Autodesk Fusion 360 part; units mm, degrees
sketch "Sketch1" plane through (0, 0, 0) normal (0, 0, 1) x (1, 0, 0)
  line L0 (-50.4372, 47.8193) -> (49.5628, 47.8193)
  line L1 (49.5628, 47.8193) -> (49.5628, -63.1807)
  line L2 (49.5628, -63.1807) -> (-50.4372, -63.1807)
  line L3 (-50.4372, -63.1807) -> (-50.4372, 47.8193)
  line L4 (-18.6372, -27.5802) -> (-23.0372, -27.5802)
  line L5 (-23.0372, -27.5802) -> (-23.0372, -24.2802)
  line L6 (-23.0372, -24.2802) -> (-18.6372, -24.2802)
  line L7 (-18.6372, -24.2802) -> (-18.6372, -27.5802)
  line L8 (17.6628, -24.0807) -> (22.0628, -24.0807)
  line L9 (22.0628, -24.0807) -> (22.0628, -27.3807)
  line L10 (22.0628, -27.3807) -> (17.6628, -27.3807)
  line L11 (17.6628, -27.3807) -> (17.6628, -24.0807)
  line L12 (17.8378, -44.4057) -> (22.2378, -44.4057)
  line L13 (22.2378, -44.4057) -> (22.2378, -47.7057)
  line L14 (22.2378, -47.7057) -> (17.8378, -47.7057)
  line L15 (17.8378, -47.7057) -> (17.8378, -44.4057)
  line L16 (27.9628, -34.1807) -> (32.3628, -34.1807)
  line L17 (32.3628, -34.1807) -> (32.3628, -37.4807)
  line L18 (32.3628, -37.4807) -> (27.9628, -37.4807)
  line L19 (27.9628, -37.4807) -> (27.9628, -34.1807)
  line L20 (-33.0372, -34.1807) -> (-28.6372, -34.1807)
  line L21 (-28.6372, -34.1807) -> (-28.6372, -37.4807)
  line L22 (-28.6372, -37.4807) -> (-33.0372, -37.4807)
  line L23 (-33.0372, -37.4807) -> (-33.0372, -34.1807)
  line L24 (-13.0372, -34.1807) -> (-8.6372, -34.1807)
  line L25 (-8.6372, -34.1807) -> (-8.6372, -37.4807)
  line L26 (-8.6372, -37.4807) -> (-13.0372, -37.4807)
  line L27 (-13.0372, -37.4807) -> (-13.0372, -34.1807)
  line L28 (-23.4439, -44.4057) -> (-19.0439, -44.4057)
  line L29 (-19.0439, -44.4057) -> (-19.0439, -47.7057)
  line L30 (-19.0439, -47.7057) -> (-23.4439, -47.7057)
  line L31 (-23.4439, -47.7057) -> (-23.4439, -44.4057)
  dimension "d1" = 100
  dimension "d2" = 111
  dimension "d3" = 4.4
  dimension "d4" = 3.3
  dimension "d5" = 4.4
  dimension "d6" = 3.3
  dimension "d7" = 4.4
  dimension "d8" = 3.3
  dimension "d9" = 4.4
  dimension "d10" = 3.3
  dimension "d11" = 4.4
  dimension "d12" = 3.3
  dimension "d13" = 4.4
  dimension "d14" = 3.3
  dimension "d15" = 4.4
  dimension "d16" = 3.3
  dimension "d17" = 17.4
  dimension "d21" = 25.7
  dimension "d22" = 25.7
  dimension "d23" = 15.475
  dimension "d24" = 15.475
  dimension "d25" = 25.7
  dimension "d26" = 27.5
  dimension "d27" = 17.2
  dimension "d28" = 15.6
  dimension "d29" = 8.656
  dimension "d30" = 8.656
  dimension "d31" = 8.656
  dimension "d32" = 35.8
  dimension "d33" = 27.325
sketch "top enclosure" plane through (0, 0, 0) normal (0, 0, 1) x (1, 0, 0)
  circle A0 centre (30.5628, -36.1807) radius 5.15
  line L0 (20.0628, -18.1807) -> (13.3583, -29.4363)
  line L1 (13.3583, -29.4363) -> (26.3583, -29.4363)
  line L2 (26.3583, -29.4363) -> (20.0628, -18.1807)
  circle A1 centre (20.0628, -46.1807) radius 5.15
  line L3 (-25.9372, -21.6807) -> (-15.9372, -21.6807)
  line L4 (-15.9372, -21.6807) -> (-15.9372, -30.6807)
  line L5 (-15.9372, -30.6807) -> (-6.9372, -30.6807)
  line L6 (-6.9372, -30.6807) -> (-6.9372, -40.6807)
  line L7 (-6.9372, -40.6807) -> (-15.9372, -40.6807)
  line L8 (-15.9372, -40.6807) -> (-15.9372, -49.6807)
  line L9 (-15.9372, -49.6807) -> (-25.9372, -49.6807)
  line L10 (-25.9372, -49.6807) -> (-25.9372, -40.6807)
  line L11 (-25.9372, -40.6807) -> (-34.9372, -40.6807)
  line L12 (-34.9372, -40.6807) -> (-34.9372, -30.6807)
  line L13 (-34.9372, -30.6807) -> (-25.9372, -30.6807)
  line L14 (-25.9372, -30.6807) -> (-25.9372, -21.6807)
  line L15 (-55.4372, 52.8193) -> (54.5628, 52.8193)
  line L16 (54.5628, 52.8193) -> (54.5628, -68.1807)
  line L17 (54.5628, -68.1807) -> (-55.4372, -68.1807)
  line L18 (-55.4372, -68.1807) -> (-55.4372, 52.8193)
  line L19 (-50.4372, -63.1807) -> (-50.4372, 47.8193)
  line L20 (49.5628, -63.1807) -> (-50.4372, -63.1807)
  line L21 (49.5628, 47.8193) -> (49.5628, -63.1807)
  line L22 (-50.4372, 47.8193) -> (49.5628, 47.8193)
  line L23 (-43.9372, 48.3193) -> (45.0628, 48.3193)
  line L24 (45.0628, 48.3193) -> (45.0628, -9.6807)
  line L25 (45.0628, -9.6807) -> (-43.9372, -9.6807)
  line L26 (-43.9372, -9.6807) -> (-43.9372, 48.3193)
  line L27 (-23.0372, -24.2802) -> (-18.6372, -24.2802)
  line L28 (-50.4372, -63.1807) -> (49.5628, -63.1807)
  line L29 (49.5628, -63.1807) -> (49.5628, 49.8193)
  line L30 (49.5628, 49.8193) -> (-50.4372, 49.8193)
  line L31 (-50.4372, 49.8193) -> (-50.4372, -63.1807)
  line L32 (44.9628, -13.6807) -> (49.5628, -13.6807)
  line L33 (49.5628, -13.6807) -> (49.5628, -23.1807)
  line L34 (49.5628, -23.1807) -> (44.9628, -23.1807)
  line L35 (44.9628, -23.1807) -> (44.9628, -13.6807)
  line L36 (-50.4372, -5.1807) -> (-36.8011, -5.1807)
  line L37 (-36.8011, -5.1807) -> (-36.8011, -27.1807)
  line L38 (-36.8011, -27.1807) -> (-50.4372, -27.1807)
  line L39 (-50.4372, -27.1807) -> (-50.4372, -5.1807)
  dimension "d34" = 60
  dimension "d35" = 10.3
  dimension "d36" = 10.3
  dimension "d37" = 10
  dimension "d38" = 10
  dimension "d39" = 10
  dimension "d40" = 10
  dimension "d41" = 9
  dimension "d42" = 9
  dimension "d43" = 9
  dimension "d44" = 9
  dimension "d45" = 9
  dimension "d46" = 9
  dimension "d47" = 13
  dimension "d49" = 11.2555
  dimension "d50" = 5
  dimension "d51" = 5
  dimension "d52" = 5
  dimension "d53" = 5
  dimension "d54" = 89
  dimension "d55" = 58
  dimension "d56" = 6.5
  dimension "d59" = 14.5995
  dimension "d60" = 45
  dimension "d61" = 27
  dimension "d62" = 17
  dimension "d63" = 13.5
  dimension "d64" = 15.5
  dimension "d65" = 19
  dimension "d66" = 29.5
  dimension "d68" = 113
  dimension "d69" = 100
  dimension "d72" = 40
  dimension "d73" = 9.5
  dimension "d74" = 4.6
  dimension "d75" = 36
  dimension "d77" = 22
extrude "Extrude6" add sketch "top enclosure" along normal blind 10 contours L15 L16 L17 L18
extrude "Extrude7" add sketch "top enclosure" along normal blind 3 contours L19 L20 L21 L22 L24 L25 L28 L29 L31 L32 L34 L35 L37 L38 | L19 L25 L26 L31 L36 L37 L38 L39 | L19 L22 L26 L31 L36 | L21 L29 L32 L33 L34 L35 | L22 L23 L24 L26 L29 L30 L31
sketch "Sketch3" plane through (54.5628, 0, 0) normal (1, 0, 0) x (0, 1, 0)
  line L0 (-68.1807, 0) -> (52.8193, 0)
  line L1 (52.8193, 0) -> (52.8193, 10)
  line L2 (52.8193, 10) -> (-68.1807, 10)
  line L3 (-68.1807, 10) -> (-68.1807, 0)
  line L4 (-18.1807, 7) -> (-8.6807, 7)
  line L5 (-8.6807, 7) -> (-8.6807, 3)
  line L6 (-8.6807, 3) -> (-18.1807, 3)
  line L7 (-18.1807, 3) -> (-18.1807, 7)
  line L8 (52.8193, 0) -> (-68.1807, 0)
  dimension "d91" = 50
  dimension "d92" = 3
  dimension "d93" = 9.5
  dimension "d94" = 4
extrude "Extrude8" cut sketch "Sketch3" against normal blind 10 contours L4 L5 L6 L7
sketch "Sketch4" plane through (49.5628, 0, 0) normal (-1, 0, 0) x (0, -1, 0)
  line L0 (8.6807, 3) -> (8.6807, 7)
  line L1 (8.6807, 7) -> (18.1807, 7)
  line L2 (18.1807, 7) -> (18.1807, 3)
  line L3 (18.1807, 3) -> (63.1807, 3)
  line L4 (63.1807, 3) -> (63.1807, 10)
  line L5 (63.1807, 10) -> (-49.8193, 10)
  line L6 (-49.8193, 10) -> (-49.8193, 3)
  line L7 (-49.8193, 3) -> (8.6807, 3)
  line L8 (7.4307, 3) -> (19.4307, 3)
  line L9 (19.4307, 3) -> (19.4307, 8.6)
  line L10 (19.4307, 8.6) -> (7.4307, 8.6)
  line L11 (7.4307, 8.6) -> (7.4307, 3)
  line L12 (8.6807, 7) -> (8.6807, 3)
  dimension "d97" = 12
  dimension "d98" = 5.6
  dimension "d99" = 1.25
extrude "Extrude9" cut sketch "Sketch4" against normal blind 2 contours L0 L1 L2 L3 L7 L8 L9 L10 L11 L12
sketch "Sketch5" plane through (-55.4372, 0, 0) normal (-1, 0, 0) x (0, -1, 0)
  line L0 (-52.8193, 0) -> (68.1807, 0)
  line L1 (68.1807, 0) -> (68.1807, 10)
  line L2 (68.1807, 10) -> (-52.8193, 10)
  line L3 (-52.8193, 10) -> (-52.8193, 0)
  line L4 (12.1807, 7.5) -> (27.1807, 7.5)
  line L5 (27.1807, 7.5) -> (27.1807, 3)
  line L6 (27.1807, 3) -> (12.1807, 3)
  line L7 (12.1807, 3) -> (12.1807, 7.5)
  dimension "d102" = 41
  dimension "d103" = 15
  dimension "d104" = 3
  dimension "d105" = 4.5
extrude "Extrude10" cut sketch "Sketch5" against normal blind 9 contours L4 L5 L6 L7
sketch "Sketch6" plane through (-50.4372, 0, 0) normal (1, 0, 0) x (0, 1, 0)
  line L0 (-27.1807, 3) -> (-27.1807, 7.5)
  line L1 (-27.1807, 7.5) -> (-12.1807, 7.5)
  line L2 (-12.1807, 7.5) -> (-12.1807, 3)
  line L3 (-12.1807, 3) -> (49.8193, 3)
  line L4 (49.8193, 3) -> (49.8193, 10)
  line L5 (49.8193, 10) -> (-63.1807, 10)
  line L6 (-63.1807, 10) -> (-63.1807, 3)
  line L7 (-63.1807, 3) -> (-27.1807, 3)
  line L8 (-28.6807, 3) -> (-10.6807, 3)
  line L9 (-10.6807, 3) -> (-10.6807, 9)
  line L10 (-10.6807, 9) -> (-28.6807, 9)
  line L11 (-28.6807, 9) -> (-28.6807, 3)
  dimension "d108" = 1.5
  dimension "d111" = 18
  dimension "d112" = 6
extrude "Extrude11" [suppressed]
Model file for the job. Use its own axes, mm. A direction names the side the tool comes from. Coordinates: 2 decimals unless noted, no trailing zeros. Order: outer loops, then holes, each group sorted by start corner. A loop starts at its lowest first (then second) coordinate and runs counter-clockwise, first axis right, second up. Notation, with made-up numbers: (87, 48.5) -> (120, 48.5) arc R8 ccw to (120, 54.5) -> close; hole circle Ø8 at (46.5, 36.25). An arc over 180 degrees is marked (long way). Return JSON: item names as keys, results as strings. Group by question number.
Item 1: Wall check: line 1 along Y through (x, z) = (-35.5, 5.75); line 2 along X through (y, z) = (-58.5, 9.25); line 3 along X through (y, z) = (-27.5, 1). Give the ranges that are in metal, low to high. Write a range as [from, to].
Item 2: Saw through at C-C on z = 5.5. Write the cut outline in (x, y).
Item 3: Pull direction Y, two halves, no side cores. Call faces 1 (the flat face through (20, -29.436, 1)), 2 (the flat face through (-11, -40.681, 1)), 3 (the flat face through (0, -68.181, 5)), 4 (the flat face through (-55.437, -9, 5)): pulls with the +Y half, pulls with the -Y half, needs draft (parallel to the pull), parting line crosses it, or undercut.
Item 4: Saw through at D-D on x = -30.5. Write the cut outline in (y, z).
Item 5: Tool access for faces 5 (the flat face through (-15.937, -26, 1)), 6 (the flat face through (53, -8.681, 5)), 7 (the flat face through (0, -63.181, 6)): list every direction of +Z, -Z, +X, -X, +Y, -Y with a clear straight run to the whole face (end or side of a thin tool).
Item 6: Saw through at A-A on x = 39. Write the cut outline in (y, z), then the cut area to 3 significant figures.
Item 7: Saw through at B-B on y = 28. Write the cut outline in (x, z), then the cut area to 3 significant figures.
Item 8: Flat gauge pin, fed straight in: P1, Ø8, axis at x = 31.5, y = -21, coming from the +Z side. Where does the tip first touch, or does it go through?
Values found:
{
 "1": {"line 1": "y = [-68.18, -63.18], [49.82, 52.82]", "line 2": "x = [-55.44, -50.44], [49.56, 54.56]", "line 3": "x = [-55.44, -25.94], [-15.94, 14.51], [25.28, 54.56]"},
 "2": {"outline": "(-55.44, -68.18) -> (54.56, -68.18) -> (54.56, -18.18) -> (51.56, -18.18) -> (51.56, -19.43) -> (49.56, -19.43) -> (49.56, -63.18) -> (-50.44, -63.18) -> (-50.44, -27.18) -> (-55.44, -27.18) -> close; (-55.44, -12.18) -> (-50.44, -12.18) -> (-50.44, 49.82) -> (49.56, 49.82) -> (49.56, -7.43) -> (51.56, -7.43) -> (51.56, -8.68) -> (54.56, -8.68) -> (54.56, 52.82) -> (-55.44, 52.82) -> close"},
 "3": {"face 1": "undercut", "face 2": "undercut", "face 3": "pulls with the -Y half", "face 4": "needs draft"},
 "4": {"outline": "(-68.18, 0) -> (-40.68, 0) -> (-40.68, 3) -> (-63.18, 3) -> (-63.18, 10) -> (-68.18, 10) -> close; (-30.68, 0) -> (-9.68, 0) -> (-9.68, 3) -> (-30.68, 3) -> close; (48.32, 0) -> (52.82, 0) -> (52.82, 10) -> (49.82, 10) -> (49.82, 3) -> (48.32, 3) -> close"},
 "5": {"face 5": "+Z, -Z", "face 6": "+X", "face 7": "+Z"},
 "6": {"outline": "(-68.18, 0) -> (-9.68, 0) -> (-9.68, 3) -> (-63.18, 3) -> (-63.18, 10) -> (-68.18, 10) -> close; (48.32, 0) -> (52.82, 0) -> (52.82, 10) -> (49.82, 10) -> (49.82, 3) -> (48.32, 3) -> close", "area": "245 mm2"},
 "7": {"outline": "(-55.44, 0) -> (-43.94, 0) -> (-43.94, 3) -> (-50.44, 3) -> (-50.44, 10) -> (-55.44, 10) -> close; (45.06, 0) -> (54.56, 0) -> (54.56, 10) -> (49.56, 10) -> (49.56, 3) -> (45.06, 3) -> close", "area": "133 mm2"},
 "8": {"P1": "stops at z = 3"}
}
